Input: part model. Units: mm. Frame: model coordinates. A direction names the side the tool comes from. Round coordinates to 2 decimals unless told otherwise and drop trailing zeros. Loops run counter-clockwise (first coordinate to the right, second up) from the corner with the lowest first, then second, coordinate; pieces in that order, holes last.
1) First-contact query: pin 1 (8 mm diameter, centred on y = 14.29, z = 41.28, fed in from +X) (3 decimals); pin 2 (11.5 mm diameter, centred on y = 14.29, z = 25.4, fed in from -X); pin 3 (8 mm diameter, centred on x = 19.5, z = 41.5, fed in from +Y) (3 decimals). Flat tips, straight axial feed; report the tip coordinate or a pass-through.
2) Ray query, line 1 along X through (y, z) = (1.65, 38.1) (3 decimals); line 2 along X through (y, z) = (9.25, 35) (3 decimals). Return the intervals inside material, ascending.
3) Access query for faces 4 (the face through (29, 3.175, 25)), 5 (the face through (17, 3, 50.8)). Directions: +Z, -Z, +X, -X, +Y, -Y. A direction counts if a zero-diameter tool reaches every point of the face in a straight line with its end or side. Return the directions, or none.
4) Section D-D, the plane y = 8.75. Return loops of the section in (x, z) (3 decimals).
5) Section A-A, the plane z = 25.4. Return loops of the section in (x, y) (1 decimal), and give its area (3 significant figures).
6) Section C-C, the plane y = 2.5. Return loops of the section in (x, z) (3 decimals), and give its area (3 significant figures).
7) Section B-B, the plane x = 41. Return loops of the section in (y, z) (3 decimals), and give its area (3 significant figures).
8) Draft query along Y for faces 1 (the face through (53.975, 2, 25)), 2 (the face through (1.57, 16.82, 9.19)), 3 (the face through (2, 28.575, 25)). Return one class per face: pulls with the +Y half, pulls with the -Y half, needs draft (parallel to the pull), parting line crosses it, or undercut.
from build123d import *

# Parameters (mm, degrees)
BOSS_EXTRUDE1_DEPTH = 50.8
SKETCH2_R           = 9.525
SKETCH2_W           = 50.8
SKETCH2_H           = 22.225
CUT_EXTRUDE1_DEPTH  = 50.8
SKETCH3_R           = 2.5527
CUT_EXTRUDE2_DEPTH  = 50.8
SKETCH4_R           = 2.5527
CUT_EXTRUDE3_DEPTH  = 3.175


with BuildPart() as part:
    # Sketch1 → Boss-Extrude1 (new body)
    with BuildSketch(Plane.XY):
        Polygon((3.175, 50.8), (0, 50.8), (0, 0), (3.175, 0), (53.975, 0), (53.975, 3.175), (3.175, 3.175), align=None)
    extrude(amount=BOSS_EXTRUDE1_DEPTH)

    # Sketch2 → Cut-Extrude1 (cut)
    with BuildSketch(Plane.ZY):
        with Locations((25.4, 14.2875)):
            Circle(SKETCH2_R)
        with Locations((25.4, 39.6875)):
            Rectangle(SKETCH2_W, SKETCH2_H)
    extrude(amount=-CUT_EXTRUDE1_DEPTH, mode=Mode.SUBTRACT)

    # Sketch3 → Cut-Extrude2 (cut)
    with BuildSketch(Plane(origin=(0, 0, 0), x_dir=(-1, 0, 0), z_dir=(0, -1, 0))):
        with Locations((-15.875, -25.4)):
            Circle(SKETCH3_R)
        with Locations((-41.275, -38.1)):
            Circle(SKETCH3_R)
        with Locations((-41.275, -12.7)):
            Circle(SKETCH3_R)
    extrude(amount=-CUT_EXTRUDE2_DEPTH, mode=Mode.SUBTRACT)

    # Sketch4 → Cut-Extrude3 (cut)
    with BuildSketch(Plane.ZY):
        with Locations((9.525, 14.2875)):
            Circle(SKETCH4_R)
        with Locations((41.275, 14.2875)):
            Circle(SKETCH4_R)
    extrude(amount=-CUT_EXTRUDE3_DEPTH, mode=Mode.SUBTRACT)


solid = part.part
Final values:
1. pin 1: stops at x = 3.175
1. pin 2: passes through
1. pin 3: stops at y = 3.175
2. line 1: x = 0 to 38.722, 43.828 to 53.975
2. line 2: x = 0 to 3.175
3. face 4: +Z, -Z, +X, +Y
3. face 5: +Z, +X, -X, +Y, -Y
4. outline: (0, 0) - (3.175, 0) - (3.175, 17.65) - (0, 17.65) - close; (0, 33.15) - (3.175, 33.15) - (3.175, 50.8) - (0, 50.8) - close
5. outline: (0, 0) - (13.3, 0) - (13.3, 3.2) - (3.2, 3.2) - (3.2, 4.8) - (0, 4.8) - close; (0, 23.8) - (3.2, 23.8) - (3.2, 28.6) - (0, 28.6) - close; (18.4, 0) - (54, 0) - (54, 3.2) - (18.4, 3.2) - close
5. area: 175 mm2
6. outline: (0, 0) - (53.975, 0) - (53.975, 50.8) - (0, 50.8) - close; hole circle Ø5.105 at (15.875, 25.4); hole circle Ø5.105 at (41.275, 12.7); hole circle Ø5.105 at (41.275, 38.1)
6. area: 2,680 mm2
7. outline: (0, 0) - (3.175, 0) - (3.175, 10.162) - (0, 10.162) - close; (0, 15.238) - (3.175, 15.238) - (3.175, 35.562) - (0, 35.562) - close; (0, 40.638) - (3.175, 40.638) - (3.175, 50.8) - (0, 50.8) - close
7. area: 129 mm2
8. face 1: needs draft
8. face 2: undercut
8. face 3: pulls with the +Y half
